Verification items for the finished model (mm, model axes). Round coordinates to 2 decimals unless told otherwise and drop trailing zeros. Loops run counter-clockwise (first coordinate to the right, second up) from the corner with the lowest first, then second, coordinate; pieces in that order, holes last. Notation, with made-up numbers: M -7,6 L 12,6 A18 ccw 12,26 Z; hole C 6.5,-16 d5. An arc over 180 degrees is marked long. Answer as CSV lines item,"result".
```python
from build123d import *

# Parameters (mm, degrees)
SKETCH5_W           = 395.4
SKETCH5_H           = 265.4
BOSS_EXTRUDE3_DEPTH = 6.35
SKETCH6_W           = 78.175
SKETCH6_H           = 243.175
SKETCH6_W_2         = 75
SKETCH6_H_2         = 240
CUT_EXTRUDE1_DEPTH  = 6.35
SKETCH10_W          = 6.35
SKETCH10_H          = 50.8
SKETCH10_W_2        = 50.8
SKETCH10_H_2        = 6.35
CUT_EXTRUDE2_DEPTH  = 6.35
SKETCH11_W          = 50.8
SKETCH11_H          = 6.35
CUT_EXTRUDE3_DEPTH  = 6.35
SKETCH12_W          = 78.175
SKETCH12_H          = 4.7625
BOSS_EXTRUDE4_DEPTH = 6.35
FILLET1_R           = 3.175
CUT_EXTRUDE4_DEPTH  = 239.190895082


with BuildPart() as part:
    # Sketch5 → Boss-Extrude3 (new body)
    with BuildSketch(Plane(origin=(0, 0, 0), x_dir=(1, 0, 0), z_dir=(0, 1, 0))):
        Rectangle(SKETCH5_W, SKETCH5_H)
    extrude(amount=BOSS_EXTRUDE3_DEPTH)

    # Sketch6 → Cut-Extrude1 (cut)
    # profile 1 of 4: a face of its own
    with BuildSketch(Plane(origin=(0, 6.35, 0), x_dir=(1, 0, 0), z_dir=(0, 1, 0))):
        with Locations((147.5, 0)):
            Rectangle(SKETCH6_W, SKETCH6_H)
        with Locations((147.5, 0)):
            Rectangle(SKETCH6_W_2, SKETCH6_H_2, mode=Mode.SUBTRACT)
    # profile 2 of 4: a face of its own
    with BuildSketch(Plane(origin=(0, 6.35, 0), x_dir=(1, 0, 0), z_dir=(0, 1, 0))):
        with Locations((147.5, 0)):
            Rectangle(SKETCH6_W_2, SKETCH6_H_2)
    # profile 3 of 4: a face of its own
    with BuildSketch(Plane(origin=(0, 6.35, 0), x_dir=(1, 0, 0), z_dir=(0, 1, 0))):
        with Locations((-147.5, 0)):
            Rectangle(SKETCH6_W, SKETCH6_H)
        with Locations((-147.5, 0)):
            Rectangle(SKETCH6_W_2, SKETCH6_H_2, mode=Mode.SUBTRACT)
    # profile 4 of 4: a face of its own
    with BuildSketch(Plane(origin=(0, 6.35, 0), x_dir=(1, 0, 0), z_dir=(0, 1, 0))):
        with Locations((-147.5, 0)):
            Rectangle(SKETCH6_W_2, SKETCH6_H_2)
    extrude(amount=-CUT_EXTRUDE1_DEPTH, mode=Mode.SUBTRACT)

    # Sketch10 → Cut-Extrude2 (cut)
    with BuildSketch(Plane.XZ):
        with Locations((98.8875, -63.5)):
            Rectangle(SKETCH10_W, SKETCH10_H)
        with Locations((98.8875, 63.5)):
            Rectangle(SKETCH10_W, SKETCH10_H)
        with Locations((-98.8875, 63.5)):
            Rectangle(SKETCH10_W, SKETCH10_H)
        with Locations((-98.8875, -63.5)):
            Rectangle(SKETCH10_W, SKETCH10_H)
        Polygon((197.7, 132.7), (177.8, 132.7), (177.8, 126.35), (191.35, 126.35), (197.7, 126.35), align=None)
        Polygon((127, 132.7), (76.2, 132.7), (76.2, 126.35), (95.7125, 126.35), (102.0625, 126.35), (108.4125, 126.35), (127, 126.35), align=None)
        with Locations((0, 129.525)):
            Rectangle(SKETCH10_W_2, SKETCH10_H_2)
        Polygon((-127, 132.7), (-127, 126.35), (-108.4125, 126.35), (-102.0625, 126.35), (-95.7125, 126.35), (-76.2, 126.35), (-76.2, 132.7), align=None)
        Polygon((-197.7, 126.35), (-191.35, 126.35), (-177.8, 126.35), (-177.8, 132.7), (-197.7, 132.7), align=None)
        Polygon((-177.8, -126.35), (-191.35, -126.35), (-197.7, -126.35), (-197.7, -132.7), (-177.8, -132.7), align=None)
        Polygon((-108.4125, -126.35), (-127, -126.35), (-127, -132.7), (-76.2, -132.7), (-76.2, -126.35), (-95.7125, -126.35), (-102.0625, -126.35), align=None)
        with Locations((0, -129.525)):
            Rectangle(SKETCH10_W_2, SKETCH10_H_2)
        Polygon((76.2, -126.35), (76.2, -132.7), (127, -132.7), (127, -126.35), (108.4125, -126.35), (102.0625, -126.35), (95.7125, -126.35), align=None)
        Polygon((177.8, -126.35), (177.8, -132.7), (197.7, -132.7), (197.7, -126.35), (191.35, -126.35), align=None)
    extrude(amount=-CUT_EXTRUDE2_DEPTH, mode=Mode.SUBTRACT)

    # Sketch11 → Cut-Extrude3 (cut)
    with BuildSketch(Plane(origin=(197.7, 0, 0), x_dir=(0, 0, -1), z_dir=(1, 0, 0))):
        with Locations((-63.5, 3.175)):
            Rectangle(SKETCH11_W, SKETCH11_H)
        with Locations((63.5, 3.175)):
            Rectangle(SKETCH11_W, SKETCH11_H)
    cut_extrude3 = extrude(amount=-CUT_EXTRUDE3_DEPTH, mode=Mode.SUBTRACT)

    # Mirror1: Cut-Extrude3 across plane
    add(cut_extrude3.mirror(Plane(origin=(0, 0, 0), x_dir=(0, 0, 1), z_dir=(1, 0, 0))), mode=Mode.SUBTRACT)

    # Sketch12 → Boss-Extrude4 (add)
    with BuildSketch(Plane.XZ):
        with Locations((147.5, -119.20625)):
            Rectangle(SKETCH12_W, SKETCH12_H)
        with Locations((147.5, 119.20625)):
            Rectangle(SKETCH12_W, SKETCH12_H)
        with Locations((-147.5, 119.20625)):
            Rectangle(SKETCH12_W, SKETCH12_H)
        with Locations((-147.5, -119.20625)):
            Rectangle(SKETCH12_W, SKETCH12_H)
    extrude(amount=-BOSS_EXTRUDE4_DEPTH)

    # Fillet1
    fillet1_edges = [part.edges().sort_by_distance(p)[0] for p in [
        (108.4125, 3.175, -116.825),
        (186.5875, 3.175, -116.825),
        (186.5875, 3.175, 116.825),
        (108.4125, 3.175, 116.825),
        (-186.5875, 3.175, 116.825),
        (-108.4125, 3.175, 116.825),
        (-108.4125, 3.175, -116.825),
        (-186.5875, 3.175, -116.825),
    ]]
    fillet(fillet1_edges, radius=FILLET1_R)

    # Sketch13 → Cut-Extrude4 (cut, through all)
    with BuildSketch(Plane.XZ):
        Polygon((69.85, 132.7), (69.85, -132.7), (76.2, -132.7), (76.2, -126.35), (127, -126.35), (127, -132.7), (177.8, -132.7), (177.8, -126.35), (197.7, -126.35), (197.7, -88.9), (191.35, -88.9), (191.35, -38.1), (197.7, -38.1), (197.7, 38.1), (191.35, 38.1), (191.35, 88.9), (197.7, 88.9), (197.7, 126.35), (177.8, 126.35), (177.8, 132.7), (127, 132.7), (127, 126.35), (76.2, 126.35), (76.2, 132.7), align=None)
        Polygon((-76.2, -132.7), (-69.85, -132.7), (-69.85, 132.7), (-76.2, 132.7), (-76.2, 126.35), (-127, 126.35), (-127, 132.7), (-177.8, 132.7), (-177.8, 126.35), (-197.7, 126.35), (-197.7, 88.9), (-191.35, 88.9), (-191.35, 38.1), (-197.7, 38.1), (-197.7, -38.1), (-191.35, -38.1), (-191.35, -88.9), (-197.7, -88.9), (-197.7, -126.35), (-177.8, -126.35), (-177.8, -132.7), (-127, -132.7), (-127, -126.35), (-76.2, -126.35), align=None)
    extrude(amount=-CUT_EXTRUDE4_DEPTH, mode=Mode.SUBTRACT)


solid = part.part
```
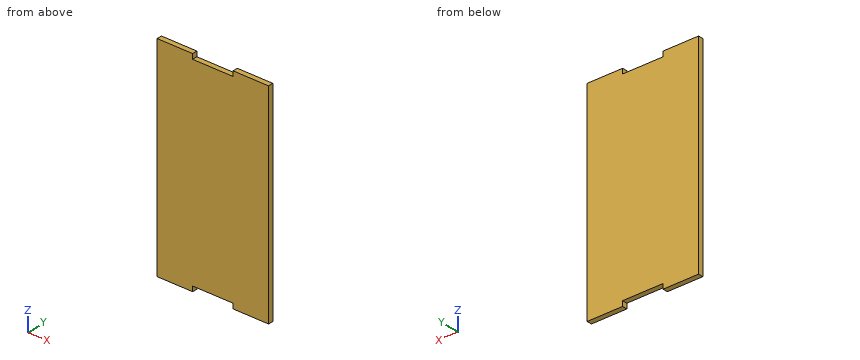
1) Material ranges on probe 1 along Z at (x, y) = (-6, 2.5), recorded low to high.
Here are the results:
probe 1,"z = -126.35 to 126.35"
2) Go/stop test with a flat-tipped pin: pin 1 (3 mm diameter, centred on x = -41.5, z = -18, fed in from -Y). Record where the tip stops, or that it passes through.
Here are the results:
pin 1,"stops at y = 0"
3) Section check A-A (y = 1). Record the cut outline in (x, z), plus the area to 3 significant figures.
Here are the results:
outline,"M -69.85,-132.7 L -25.4,-132.7 L -25.4,-126.35 L 25.4,-126.35 L 25.4,-132.7 L 69.85,-132.7 L 69.85,132.7 L 25.4,132.7 L 25.4,126.35 L -25.4,126.35 L -25.4,132.7 L -69.85,132.7 Z"
area,"36,400 mm^2"
4) Section check B-B (x = -8). Record the cut outline in (y, z).
Here are the results:
outline,"M 0,-126.35 L 6.35,-126.35 L 6.35,126.35 L 0,126.35 Z"
